Model file for the job. Use its own axes, mm. A direction names the side the tool comes from. Round coordinates to 2 decimals unless told otherwise and drop trailing zeros. Loops run counter-clockwise (first coordinate to the right, second up) from the corner with the lowest first, then second, coordinate; pieces in that order, holes last. Notation, with made-up numbers: M 24,1 L 66,1 A20 cw 66,27 Z; hole C 31.5,55 d10. An arc over 180 degrees is marked long. Answer in a Markdown table with one row per item.
Autodesk Inventor part; units mm, degrees
ref_plane "YZ Plane" through (0, 0, 0) normal (1, 0, 0) x (0, 1, 0)
ref_plane "XZ Plane" through (0, 0, 0) normal (0, 1, 0) x (-1, 0, 0)
ref_plane "XY Plane" through (0, 0, 0) normal (0, 0, 1) x (1, 0, 0)
sketch "草圖1" plane through (0, 0, 0) normal (0, 0, 1) x (1, 0, 0)
  line L0 (0, 0) -> (20, 0)
  line L1 (20, 0) -> (20, 10)
  line L2 (20, 10) -> (10, 45)
  line L3 (12, 47) -> (10, 45)
  line L4 (12, 47) -> (12, 54)
  line L5 (11, 55) -> (0, 55)
  line L6 (12, 54) -> (11, 55)
  line L7 (0, 0) -> (0, 55)
  point P0 (12, 55)
  dimension "d0" = 20
  dimension "d1" = 10
  dimension "d4" = 8
  dimension "d5" = 1
  dimension "d6" = 45
  dimension "d7" = 2
  dimension "d8" = 2
  dimension "d9" = 55
  dimension "d10" = 10
revolve "迴轉1" add sketch "草圖1" angle 360 about axis through (0, 0, 0) along (0, 1, 0)
sketch "草圖2" plane through (0, 0, 0) normal (0, 0, 1) x (1, 0, 0)
  line L0 (0, 0) -> (15, 0)
  line L1 (-20, 0) -> (20, 0)
  line L2 (15, 0) -> (6, 33)
  line L3 (6, 33) -> (0, 33)
  line L4 (0, 33) -> (0, 0)
  dimension "d12" = 15
  dimension "d13" = 6
  dimension "d14" = 33
revolve "迴轉2" cut sketch "草圖2" angle 360 about axis through (0, 33, 0) along (0, -1, 0)
sketch "草圖3" plane through (0, 33, 0) normal (0, -1, 0) x (1, 0, 0)
  circle A0 centre (0, 0) radius 6
  dimension "d16" = 12
extrude "擠出1" cut sketch "草圖3" against normal through all
thread "螺紋1"
properties part number "C"
1. Saw through at D-D (y = 9). Write the cut outline in (x, z), and give its area (3 significant figures).
Verdict:
| item | result |
|---|---|
| outline | C 0,0 d40; hole C 0,0 d25.09 |
| area | 762 mm² |
2. Saw through at C-C (y = 50). Write the cut outline in (x, z), and give its area (3 significant figures).
Verdict:
| item | result |
|---|---|
| outline | C 0,0 d24; hole C 0,0 d12 |
| area | 339 mm² |
3. Pin check, flat tips, straight feed: pin 1 (4 mm diameter, centred on y = 46.5, z = -8.5, fed in from -X); pin 2 (11 mm diameter, centred on x = 0, z = 0, fed in from +Y); pin 3 (5 mm diameter, centred on y = 16.5, z = 4, fed in from -X); pin 4 (3 mm diameter, centred on x = -5.5, y = 42, fed in from +Z). Stop position of each tip, or through.
Verdict:
| item | result |
|---|---|
| pin 1 | stops at x = -10.05 |
| pin 2 | passes through |
| pin 3 | stops at x = -18.56 |
| pin 4 | stops at z = 10.25 |
4. Tool access for faces 1 (the cylindrical face through (-11.99, 50.55, -0.53)), 2 (the conical face through (-1.318, 45.125, -10.039)), 3 (the flat face through (3, 0, -15)): list every direction of +Z, -Z, +X, -X, +Y, -Y with a clear straight run to the whole face (end or side of a thin tool).
Verdict:
| item | result |
|---|---|
| face 1 | +Y |
| face 2 | none |
| face 3 | +Z, -Z, +X, -X, -Y |
5. Mould opens along X. For faces 4 (the cylindrical face through (-6, 44, 0)), 5 (the flat face through (5, 55, 5)), 6 (the conical face through (-7.589, 19.936, -5.819)), 7 (the conical face through (-3.026, 31.144, -13.627)) say: +X half, -X half, draft (parallel to the pull), parting line (faces both ways), or undercut.
Verdict:
| item | result |
|---|---|
| face 4 | undercut |
| face 5 | draft |
| face 6 | undercut |
| face 7 | parting line |
6. Wall check: probe 1 along Z at (x, y) = (0, 38); probe 2 along Z at (x, y) = (-0.5, 16.5); probe 3 along X at (y, z) = (26, -2). Give the ranges that are in metal, low to high.
Verdict:
| item | result |
|---|---|
| probe 1 | z = -12 to -6, 6 to 12 |
| probe 2 | z = -18.14 to -10.49, 10.49 to 18.14 |
| probe 3 | x = -15.3 to -7.65, 7.65 to 15.3 |
7. Saw through at A-A (x = 0). Write the cut outline in (y, z).
Verdict:
| item | result |
|---|---|
| outline | M 0,-20 L 10,-20 L 45,-10 L 47,-12 L 54,-12 L 55,-11 L 55,-6 L 33,-6 L 0,-15 Z; M 0,15 L 33,6 L 55,6 L 55,11 L 54,12 L 47,12 L 45,10 L 10,20 L 0,20 Z |
8. Saw through at B-B (z = 0). Write the cut outline in (x, y), and give its area (3 significant figures).
Verdict:
| item | result |
|---|---|
| outline | M -20,0 L -15,0 L -6,33 L -6,55 L -11,55 L -12,54 L -12,47 L -10,45 L -20,10 Z; M 6,33 L 15,0 L 20,0 L 20,10 L 10,45 L 12,47 L 12,54 L 11,55 L 6,55 Z |
| area | 728 mm² |
